Print and shaded views of the part. All mm, measured from the part's lowest x, y and z. A direction names the side the tool comes from. Coordinates: 2 decimals unless noted, no trailing zeros. Order: outer loops, then holes, each group sorted by start corner. A loop starts at its lowest first (then second) coordinate and runs counter-clockwise, first axis right, second up. Notation, with made-up numbers: M 11,49.25 L 28,49.25 A19 cw 28,69.25 Z; hole C 67.5,55 d9. An arc over 180 degrees is marked long. Return JSON: item names as keys, results as strings.
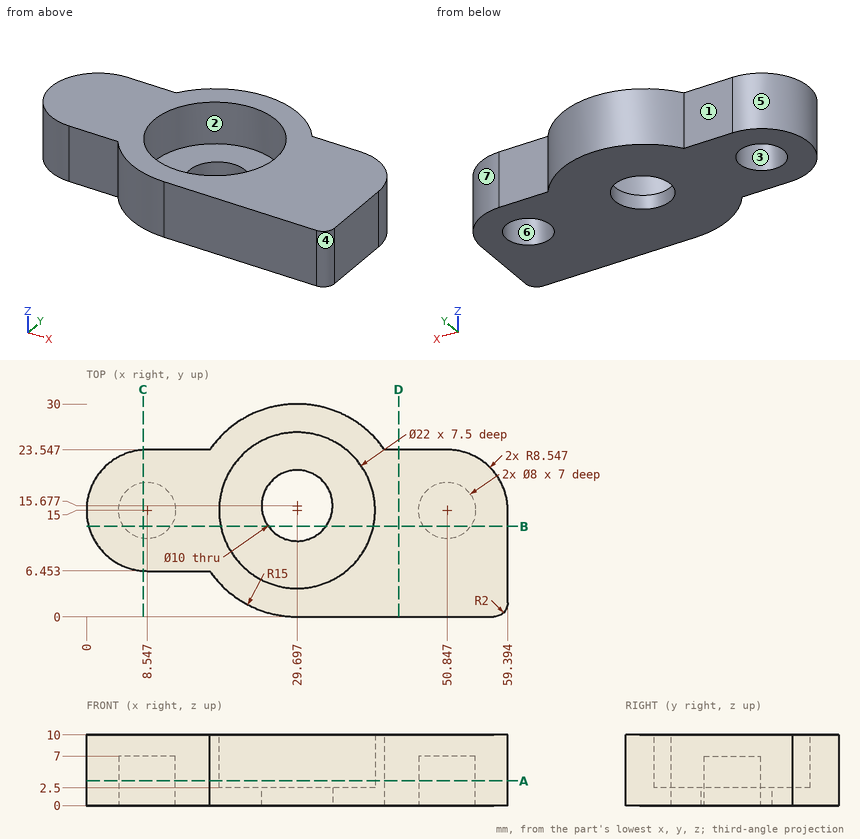
Item 1: Saw through at C-C (x = 8). Write the cut outline in (y, z), and give its area (3 significant figures).
Check result:
{"outline": "M 6.47,0 L 11.04,0 L 11.04,7 L 18.96,7 L 18.96,0 L 23.53,0 L 23.53,10 L 6.47,10 Z", "area": "115 mm2"}
Item 2: Pull direction Y, two halves, no side cores. Call the marked faces 4, 5, 6 and 7: +Y half, -Y half, draft (parallel to the pull), parting line (faces both ways), or undercut.
Check result:
{"face 4": "-Y half", "face 5": "parting line", "face 6": "undercut", "face 7": "+Y half"}
Item 3: Wall check: line 1 (Z direction, x = 52, y = 17.75); line 2 (Y direction, x = 25, z = 3) (1 decimal); line 3 (Y direction, x = 27.5, z = 4.25). Give the ranges that are in metal, low to high.
Check result:
{"line 1": "z = 7 to 10", "line 2": "y = 0.8 to 5.1, 24.9 to 29.2", "line 3": "y = 0.16 to 4.22, 25.78 to 29.84"}
Item 4: Saw through at A-A (z = 3.5). Write the cut outline in (x, y).
Check result:
{"outline": "M 8.55,6.45 L 17.37,6.45 A15 ccw 29.7,0 L 57.39,0 A2 ccw 59.39,2 L 59.39,15 A8.55 ccw 50.85,23.55 L 42.02,23.55 A15 ccw 17.37,23.55 L 8.55,23.55 A8.55 ccw Z; hole C 8.55,15 d8; hole C 29.7,15 d22; hole C 50.85,15 d8"}
Item 5: Saw through at D-D (x = 44). Write the cut outline in (y, z).
Check result:
{"outline": "M 0,0 L 23.55,0 L 23.55,10 L 0,10 Z"}
Item 6: Drop flat-ended pins along their axis: pin 1 Ø4.5 at (x, z) = (47.5, 3.5) entering from +Y; pin 2 Ø6 at (x, y) = (35, 11) entering from +Z; pin 3 Ø6 at (x, z) = (25, 2) entering from -Y; pin 4 Ø6 at (x, y) = (29.7, 15.68) entering from +Z. Give the stop position or say it passes through.
Check result:
{"pin 1": "stops at y = 23.55", "pin 2": "stops at z = 2.5", "pin 3": "stops at y = 0.1", "pin 4": "passes through"}
Item 7: 3-axis set-ups, long thin cutter, end or side, ignore diameter. For the marked faces 1, 2 and 3: which of +Z, -Z, +X, -X, +Y, -Y reach the whole face in a straight line?
Check result:
{"face 1": "+Z, -Z, -X, +Y", "face 2": "+Z", "face 3": "-Z"}
Item 8: Saw through at B-B (y = 12.75). Write the cut outline in (x, z) (1 decimal).
Check result:
{"outline": "M 0.3,0 L 5.2,0 L 5.2,7 L 11.9,7 L 11.9,0 L 25.6,0 L 25.6,2.5 L 18.9,2.5 L 18.9,10 L 0.3,10 Z; M 33.8,0 L 47.5,0 L 47.5,7 L 54.2,7 L 54.2,0 L 59.4,0 L 59.4,10 L 40.5,10 L 40.5,2.5 L 33.8,2.5 Z"}
